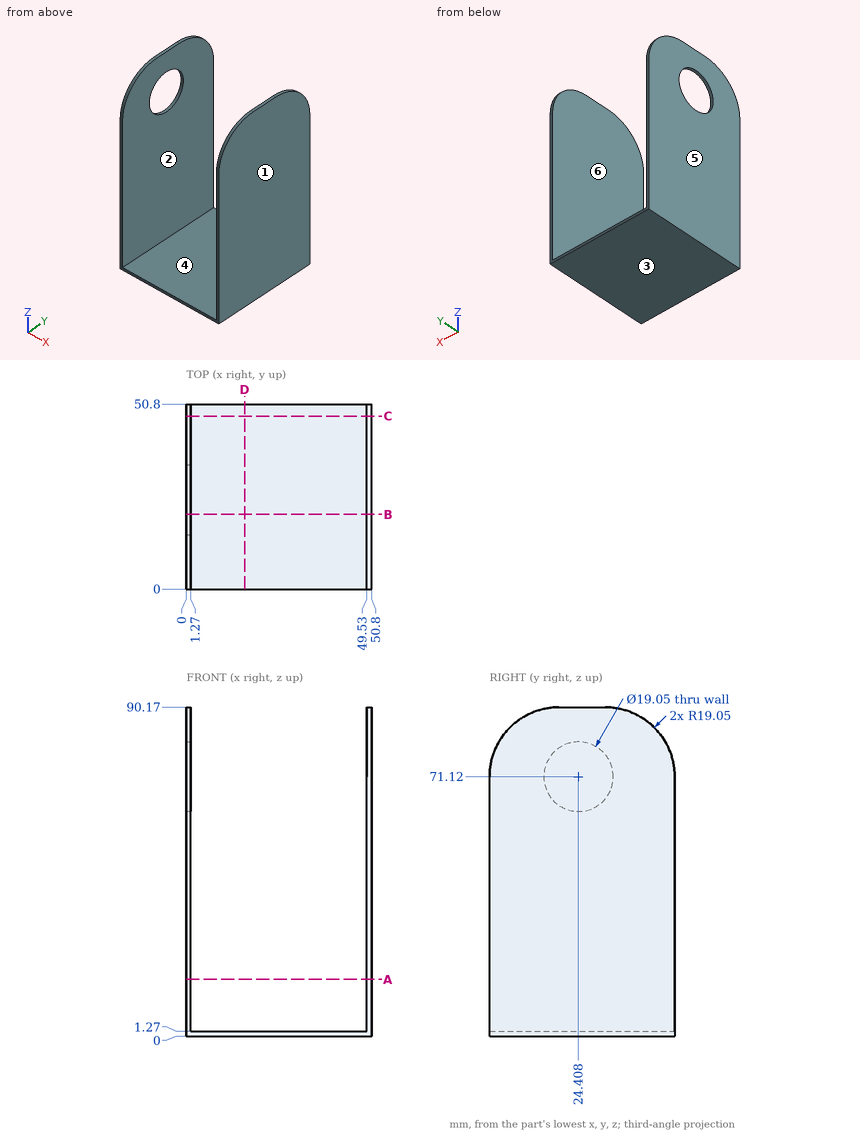
Design review of the part shown in the three views and the two pictorial views. Dimensions are in mm from the part's minimum x, y and z. A direction names the side the tool comes from. Round coordinates to 2 decimals unless told otherwise and drop trailing zeros. Loops run counter-clockwise (first coordinate to the right, second up) from the corner with the lowest first, then second, coordinate; pieces in that order, holes last. Notation, with made-up numbers: (-25, 61.5) -> (-1, 61.5) arc R21 cw to (-1, 75.5) -> close; hole circle Ø1 at (3, -13.5). An arc over 180 degrees is marked (long way). Answer as a JSON object with one key per item and string values. Group by question number.
1) We need section B-B on y = 20.5. Write out the cut boundary in (x, z), then the cut area to 3 significant figures.
2) We need section A-A on z = 15.5. Write out the cut boundary in (x, y).
3) We need section D-D on x = 16. Write out the cut boundary in (y, z).
4) For line 1 (X direction, y = 38, z = 52); line 2 (Z direction, x = 24, y = 14), list the stretches that pass through material, from the lowest coordinate up. Write a range as [from, to].
5) For pin 1 Ø1.5 at (x, y) = (30, 28.5) entering from +Z; pin 2 Ø11.5 at (y, z) = (24.41, 71.12) entering from -X, all flat-tipped, find the tip position at first contact; note any pin that passes through.
6) For the marked faces 1 and 2, list the 3-axis set-ups (+Z, -Z, +X, -X, +Y, -Y) from which the entire face can be reached by the end or side of a thin tool; tool diameter is ignored.
7) We need section C-C on y = 47.5. Write out the cut boundary in (x, z).
8) Mouldability with a two-part tool opening along X and no side actions: class the marked faces 3, 4, 5 and 6 as released by +X, released by -X, zero draft, split by the parting line, or undercut.
Result set:
{
 "1": {"outline": "(0, 0) -> (50.8, 0) -> (50.8, 90.17) -> (49.53, 90.17) -> (49.53, 1.27) -> (1.27, 1.27) -> (1.27, 62.43) -> (0, 62.43) -> close; (0, 79.81) -> (1.27, 79.81) -> (1.27, 90.17) -> (0, 90.17) -> close", "area": "268 mm²"},
 "2": {"outline": "(0, 0) -> (1.27, 0) -> (1.27, 50.8) -> (0, 50.8) -> close; (49.53, 0) -> (50.8, 0) -> (50.8, 50.8) -> (49.53, 50.8) -> close"},
 "3": {"outline": "(0, 0) -> (50.8, 0) -> (50.8, 1.27) -> (0, 1.27) -> close"},
 "4": {"line 1": "[0, 1.27], [49.53, 50.8]", "line 2": "[0, 1.27]"},
 "5": {"pin 1": "z = 1.27", "pin 2": "x = 49.53"},
 "6": {"face 1": "+Z, -Z, +X, +Y, -Y", "face 2": "+Z, +Y, -Y"},
 "7": {"outline": "(0, 0) -> (50.8, 0) -> (50.8, 81.84) -> (49.53, 81.84) -> (49.53, 1.27) -> (1.27, 1.27) -> (1.27, 81.84) -> (0, 81.84) -> close"},
 "8": {"face 3": "zero draft", "face 4": "undercut", "face 5": "released by -X", "face 6": "undercut"}
}
